Geometry: final body of the model. Coordinates: model frame, mm. Coordinates: 2 decimals unless noted, no trailing zeros. Write each loop counter-clockwise with the first axis right and the second up, starting at its lowest first coordinate (ties: lowest second). Pieces come first, ordered by that corner, then holes.
from build123d import *

# Parameters (mm, degrees)
SKETCH_1_W          = 100
SKETCH_1_H          = 15
SKETCH_1_R          = 3
SKETCH_1_R_2        = 5.021699513
EXTRUDE_1_DEPTH     = 15
CUT_EXTRUDE_1_REACH = 94.083
SKETCH_2_R          = 3


with BuildPart() as part:
    # 草圖1 → 填料-伸長1 (new body)
    with BuildSketch(Plane.XY):
        with Locations((39.606552155, 35.683485423)):
            Rectangle(SKETCH_1_W, SKETCH_1_H)
        with Locations((82.106552155, 35.683485423)):
            Circle(SKETCH_1_R, mode=Mode.SUBTRACT)
        with Locations((-2.893447845, 35.683485423)):
            Circle(SKETCH_1_R_2, mode=Mode.SUBTRACT)
    extrude(amount=EXTRUDE_1_DEPTH)

    # 草圖2 → 除料-伸長1 (cut, up to next)
    with BuildSketch(Plane.XZ.offset(-28.183485423), mode=Mode.PRIVATE) as cut_extrude_1_sk1:
        with Locations((60.806805045, 7.5)):
            Circle(SKETCH_2_R)
    cut_extrude_1_tool1 = extrude(cut_extrude_1_sk1.sketch, amount=-CUT_EXTRUDE_1_REACH, mode=Mode.PRIVATE) & part.part
    # 草圖2 → 除料-伸長1 (cut, up to next)
    with BuildSketch(Plane.XZ.offset(-28.183485423), mode=Mode.PRIVATE) as cut_extrude_1_sk2:
        with Locations((25.293048558, 7.5)):
            Circle(SKETCH_2_R)
    cut_extrude_1_tool2 = extrude(cut_extrude_1_sk2.sketch, amount=-CUT_EXTRUDE_1_REACH, mode=Mode.PRIVATE) & part.part
    add(cut_extrude_1_tool1.solids().sort_by_distance((60.806805, 28.183485, 7.5))[0], mode=Mode.SUBTRACT)
    add(cut_extrude_1_tool2.solids().sort_by_distance((25.293049, 28.183485, 7.5))[0], mode=Mode.SUBTRACT)


solid = part.part
Item 1: Pull-direction query (Y, two-part tool) for faces 1 (the cylindrical face through (79.11, 35.82, 7.4)), 2 (the flat face through (39, 28.183, 7)), 3 (the flat face through (39, 36, 15)); classes: released by +Y, released by -Y, zero draft, split by the parting line, or undercut.
Derived:
face 1: undercut
face 2: released by -Y
face 3: zero draft
Item 2: Section B-B, the plane z = 7.5. Output: boundary loops of the cut face in (x, y), plus the area to 3 significant figures.
Derived:
outline: (-10.39, 28.18) - (22.29, 28.18) - (22.29, 43.18) - (-10.39, 43.18) - close; (28.29, 28.18) - (57.81, 28.18) - (57.81, 43.18) - (28.29, 43.18) - close; (63.81, 28.18) - (89.61, 28.18) - (89.61, 43.18) - (63.81, 43.18) - close; hole circle Ø10.04 at (-2.89, 35.68); hole circle Ø6 at (82.11, 35.68)
area: 1,210 mm2
Item 3: Section C-C, the plane x = -3. Output: boundary loops of the cut face in (y, z), plus the area to 3 significant figures.
Derived:
outline: (28.18, 0) - (30.66, 0) - (30.66, 15) - (28.18, 15) - close; (40.7, 0) - (43.18, 0) - (43.18, 15) - (40.7, 15) - close
area: 74.4 mm2
Item 4: Pin query (flat end, axial travel): pin 1 (8 mm diameter, centred on x = -2.89, y = 35.68, fed in from -Z); pin 2 (1.5 mm diameter, centred on x = 58.5, y = 35.5, fed in from -Z). Return the tip coordinate at first contact, or that it passes through.
Derived:
pin 1: passes through
pin 2: stops at z = 0
Item 5: Section A-A, the plane y = 33.75. Output: boundary loops of the cut face in (x, z), plus the area to 3 significant figures.
Derived:
outline: (-10.39, 0) - (-7.53, 0) - (-7.53, 15) - (-10.39, 15) - close; (1.74, 0) - (79.81, 0) - (79.81, 15) - (1.74, 15) - close; (84.4, 0) - (89.61, 0) - (89.61, 15) - (84.4, 15) - close; hole circle Ø6 at (25.29, 7.5); hole circle Ø6 at (60.81, 7.5)
area: 1,240 mm2
Item 6: Material intervals for probe 1 along X at (y, z) = (30.25, 5.25); probe 2 along X at (y, z) = (31.25, 10); probe 3 along X at (y, z) = (29.5, 9.5), sorted ascending.
Derived:
probe 1: x = -10.39 to 23.31, 27.28 to 58.82, 62.79 to 89.61
probe 2: x = -10.39 to -5.25, -0.54 to 23.63, 26.95 to 59.15, 62.47 to 89.61
probe 3: x = -10.39 to 23.06, 27.53 to 58.57, 63.04 to 89.61
